from build123d import *

# Parameters (mm, degrees)
SKETCH1_W           = 10
SKETCH1_H           = 6
SKETCH1_R           = 0.75
BOSS_EXTRUDE1_DEPTH = 2
SKETCH2_W           = 10
SKETCH2_H           = 6
SKETCH2_R           = 0.75
BOSS_EXTRUDE2_DEPTH = 2
FILLET2_R           = 2.5


with BuildPart() as part:
    # Sketch1 → Boss-Extrude1 (new body)
    with BuildSketch(Plane.XY):
        with Locations((-5, -3)):
            Rectangle(SKETCH1_W, SKETCH1_H)
        with Locations((-3, -3)):
            Circle(SKETCH1_R, mode=Mode.SUBTRACT)
    extrude(amount=BOSS_EXTRUDE1_DEPTH)

    # Sketch2 → Boss-Extrude2 (add)
    with BuildSketch(Plane.ZY.offset(10)):
        with Locations((5, -3)):
            Rectangle(SKETCH2_W, SKETCH2_H)
        with Locations((5.9, -2.4)):
            Circle(SKETCH2_R, mode=Mode.SUBTRACT)
    extrude(amount=-BOSS_EXTRUDE2_DEPTH)

    # Fillet2
    fillet2_edges = [part.edges().sort_by_distance(p)[0] for p in [
        (-8, -3, 2),
    ]]
    fillet(fillet2_edges, radius=FILLET2_R)


solid = part.part
Design review of the part built by this model. Coordinates are the model's own, in mm. A direction names the side the tool comes from. Coordinates: 2 decimals unless noted, no trailing zeros. Loops run counter-clockwise (first coordinate to the right, second up) from the corner with the lowest first, then second, coordinate; pieces in that order, holes last.
Item 1: Draft analysis for pull direction X (two halves, no side actions). For faces 3 (the cylindrical face through (-3.595, -3.456, 0.986)), 4 (the flat face through (-2, -3, 2)), 5 (the flat face through (0, -3, 1)), state which applies: pulls with the +X half, pulls with the -X half, needs draft (parallel to the pull), parting line crosses it, or undercut.
Completed:
face 3: undercut
face 4: needs draft
face 5: pulls with the +X half
Item 2: Add section B-B (x = -3). Write out the cut boundary in (y, z), and give its area (3 significant figures).
Completed:
outline: (-6, 0) - (-3.75, 0) - (-3.75, 2) - (-6, 2) - close; (-2.25, 0) - (0, 0) - (0, 2) - (-2.25, 2) - close
area: 9.00 mm2
Item 3: Add section C-C (z = 5.5). Write out the cut boundary in (x, y), and give its area (3 significant figures).
Completed:
outline: (-10, -6) - (-8, -6) - (-8, -3.03) - (-10, -3.03) - close; (-10, -1.77) - (-8, -1.77) - (-8, 0) - (-10, 0) - close
area: 9.46 mm2
Item 4: Add section A-A (y = -3). Write out the cut boundary in (x, z), and give its area (3 significant figures).
Completed:
outline: (-10, 0) - (-3.75, 0) - (-3.75, 2) - (-5.5, 2) arc R2.5 cw to (-8, 4.5) - (-8, 5.45) - (-10, 5.45) - close; (-10, 6.35) - (-8, 6.35) - (-8, 10) - (-10, 10) - close; (-2.25, 0) - (0, 0) - (0, 2) - (-2.25, 2) - close
area: 32.5 mm2
Item 5: Wall thickness on L1, parallel to Y at x = -3, z = 1.15; L2, parallel to Y at x = -9.5, z = 5.9; L3, parallel to X at y = -2.15, z = 8: over which ranges is each line inside the solid? List them lowest first.
Completed:
L1: y = -6 to -3.75, -2.25 to 0
L2: y = -6 to -3.15, -1.65 to 0
L3: x = -10 to -8
Item 6: Clearance check with flat-ended pins moving along their axes: pin 1 (1.6 mm diameter, centred on x = -2, y = -2, fed in from +Z); pin 2 (3 mm diameter, centred on x = -5, z = 8.5, fed in from -Y); pin 3 (1.6 mm diameter, centred on y = -3.5, z = 7.5, fed in from +X). State where each tip first meets the part, or that it passes through.
Completed:
pin 1: stops at z = 2
pin 2: passes through
pin 3: stops at x = -8
Item 7: Add section D-D (x = -8.75). Write out the cut boundary in (y, z).
Completed:
outline: (-6, 0) - (0, 0) - (0, 10) - (-6, 10) - close; hole circle Ø1.5 at (-2.4, 5.9)
Item 8: For faces 1 (the cylindrical face through (-9.014, -2.175, 6.615)), 2 (the flat face through (-8, -3, 7)), list the 3-axis set-ups (+Z, -Z, +X, -X, +Y, -Y) from which the entire face can be reached by the end or side of a thin tool; tool diameter is ignored.
Completed:
face 1: +X, -X
face 2: +Z, +X, +Y, -Y
